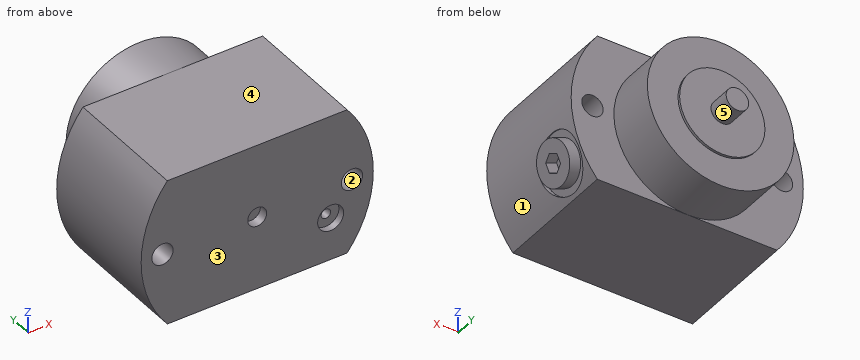
from build123d import *

# Parameters (mm, degrees)
EXTRUDE1_DEPTH     = 53
HOLE1_D            = 9
HOLE1_DEPTH        = 53
SKETCH5_R          = 4
CUT_EXTRUDE1_DEPTH = 4
SKETCH6_R          = 5.5
CUT_EXTRUDE2_DEPTH = 3
SKETCH7_R          = 2
CUT_EXTRUDE3_DEPTH = 33
CUT_EXTRUDE4_DEPTH = 5


with BuildPart() as part:
    # Sketch1 → Extrude1 (new body)
    with BuildSketch(Plane(origin=(0, 0, 0), x_dir=(1, 0, 0), z_dir=(0, 1, 0))):
        with BuildLine():
            Line((-37.947331922, 31), (37.947331922, 31))
            ThreePointArc((37.947331922, 31), (49, 0), (37.947331922, -31))
            Line((37.947331922, -31), (-37.947331922, -31))
            ThreePointArc((-37.947331922, -31), (-49, 0), (-37.947331922, 31))
        make_face()
    extrude(amount=EXTRUDE1_DEPTH)

    # Sketch2 → Revolve1 (revolve)
    with BuildSketch(Plane.XY, mode=Mode.PRIVATE) as revolve1_sk:
        Polygon((0, 84.5), (-4.75, 84.5), (-4.75, 75), (-18, 75), (-18, 74), (-30.95, 74), (-30.95, 53), (0, 53), align=None)
    revolve(revolve1_sk.sketch.rotate(Axis((0, 0, 0), (0, 1, 0)), 270), axis=Axis((0, 0, 0), (0, 1, 0)))  # turned: the seam where the file's is

    # Hole1
    with Locations(Plane(origin=(0, 53, 0), x_dir=(-1, 0, 0), z_dir=(0, 1, 0))):
        with Locations((40, 0), (-40, 0)):
            Hole(HOLE1_D / 2, depth=HOLE1_DEPTH)

    # Sketch5 → Cut-Extrude1 (cut)
    with BuildSketch(Plane.XZ):
        with Locations(Location((0, 0, 0), (0, 0, 270))):  # turned: the seam where the file's is
            Circle(SKETCH5_R)
    extrude(amount=-CUT_EXTRUDE1_DEPTH, mode=Mode.SUBTRACT)

    # Sketch6 → Cut-Extrude2 (cut)
    with BuildSketch(Plane.XZ):
        with Locations(Location((31, -13, 0), (0, 0, 270))):  # turned: the seam where the file's is
            Circle(SKETCH6_R)
    extrude(amount=-CUT_EXTRUDE2_DEPTH, mode=Mode.SUBTRACT)

    # Sketch7 → Cut-Extrude3 (cut)
    with BuildSketch(Plane.XZ.offset(-3)):
        with Locations(Location((31, -13, 0), (0, 0, 270))):  # turned: the seam where the file's is
            Circle(SKETCH7_R)
    extrude(amount=-CUT_EXTRUDE3_DEPTH, mode=Mode.SUBTRACT)

    # Sketch8 → Cut-Revolve1 (revolve, cut)
    with BuildSketch(Plane(origin=(0, 0, 0), x_dir=(0.920504853, 0, -0.390731128), z_dir=(0.390731128, 0, 0.920504853)), mode=Mode.PRIVATE) as cut_revolve1_sk:
        Polygon((49, 28), (47, 28), (47, 33.4215), (45.517364509, 34.2775), (32, 34.2775), (32, 40), (49, 40), align=None)
    revolve(cut_revolve1_sk.sketch.rotate(Axis((47.484793311, 40, -20.156098913), (-0.920504853, 0, 0.390731128)), 270), axis=Axis((47.484793311, 40, -20.156098913), (-0.920504853, 0, 0.390731128)), mode=Mode.SUBTRACT)  # turned: the seam where the file's is

    # Sketch9 → Revolve2 (revolve)
    with BuildSketch(Plane(origin=(0, 0, 0), x_dir=(0.920504853, 0, -0.390731128), z_dir=(0.390731128, 0, 0.920504853)), mode=Mode.PRIVATE) as revolve2_sk:
        Polygon((47, 31), (47, 34.2775), (38, 34.2775), (37, 35.2775), (37, 40), (52, 40), (52, 31), align=None)
    revolve(revolve2_sk.sketch.rotate(Axis((53.930450878, 40, -22.892118224), (-0.920504853, 0, 0.390731128)), 270), axis=Axis((53.930450878, 40, -22.892118224), (-0.920504853, 0, 0.390731128)))  # turned: the seam where the file's is

    # Sketch10 → Cut-Extrude4 (cut)
    with BuildSketch(Plane(origin=(47.86625238, 0, -20.318018681), x_dir=(-0.390731128, 0, -0.920504853), z_dir=(0.920504853, 0, -0.390731128))):
        Polygon((4.041451884, 40), (2.020725942, 43.5), (-2.020725942, 43.5), (-4.041451884, 40), (-2.020725942, 36.5), (2.020725942, 36.5), align=None)
    extrude(amount=-CUT_EXTRUDE4_DEPTH, mode=Mode.SUBTRACT)


solid = part.part
CAD build for the part. Positions are in the model's coordinates, mm. Face numbers are marked on the shaded views. A direction names the side the tool comes from. Round coordinates to 2 decimals unless told otherwise and drop trailing zeros. Order: outer loops, then holes, each group sorted by start corner. A loop starts at its lowest first (then second) coordinate and runs counter-clockwise, first axis right, second up. Notation, with made-up numbers: (82.5, 68) -> (132.5, 68) arc R9 ccw to (132.5, 84) -> close; hole circle Ø1 at (6, 66). An arc over 180 degrees is marked (long way). Write item = value, one per line. Start each with the question number.
(1) Probe line 1 (X direction, y = 19, z = 0.5); line 2 (X direction, y = 81, z = 0); line 3 (Y direction, x = 29, z = 23.5). List the from-to ranges inside material, lowest first. Write a range as [from, to].
(2) Cut at D-D, the plane x = 0. List the corners of the cut face in (y, z), then the cut area to 3 significant figures.
(3) Pin check, flat tips, straight feed: P1, Ø0.8, axis at x = 29.5, z = -12, coming from the -Y side; P2, Ø8, axis at x = 40, z = 0, coming from the -Y side; P3, Ø3, axis at x = 31, z = -13, coming from the -Y side; P4, Ø6, axis at x = 11.5, z = -13.5, coming from the +Y side. Stop position of each tip, or through.
(4) Which spindle directions (+Z, -Z, +X, -X, +Y, -Y) get a long thin tool onto all of the face, cutting with end or side? Do the marked faces 4 and 5. Say none if no direction does.
(5) Pull direction X, two halves, no side cores. Call the marked faces 1, 2 and 3: released by +X, released by -X, zero draft, split by the parting line, or undercut.
(6) Cut at B-B, the plane x = -40. List the corners of the cut face in (y, z), then the cut area to 3 significant figures.
(7) Cut at A-A, the plane z = 0. List the corners of the cut face in (x, y), then the cut area to 3 significant figures.
(8) Cut at C-C, the plane y = 11.5. List the corners of the cut face in (x, z).
Model answer:
q1.line_1 = [-49, -44.47], [-35.53, 35.53], [44.47, 49]
q1.line_2 = [-4.75, 4.75]
q1.line_3 = [0, 53]
q2.outline = (0, -31) -> (53, -31) -> (53, -30.95) -> (74, -30.95) -> (74, -18) -> (75, -18) -> (75, -4.75) -> (84.5, -4.75) -> (84.5, 4.75) -> (75, 4.75) -> (75, 18) -> (74, 18) -> (74, 30.95) -> (53, 30.95) -> (53, 31) -> (0, 31) -> (0, 4) -> (4, 4) -> (4, -4) -> (0, -4) -> close
q2.area = 4,680 mm2
q3.P1 = 3
q3.P2 = through
q3.P3 = 45.48
q3.P4 = 75
q4.face_4 = +Z, +X, -X, +Y, -Y
q4.face_5 = +Y
q5.face_1 = released by +X
q5.face_2 = undercut
q5.face_3 = zero draft
q6.outline = (0, -28.3) -> (53, -28.3) -> (53, -4.5) -> (0, -4.5) -> close; (0, 4.5) -> (53, 4.5) -> (53, 28.3) -> (0, 28.3) -> close
q6.area = 2,520 mm2
q7.outline = (-49, 0) -> (-44.5, 0) -> (-44.5, 53) -> (-49, 53) -> close; (-35.5, 0) -> (-4, 0) -> (-4, 4) -> (4, 4) -> (4, 0) -> (35.5, 0) -> (35.5, 53) -> (30.95, 53) -> (30.95, 74) -> (18, 74) -> (18, 75) -> (4.75, 75) -> (4.75, 84.5) -> (-4.75, 84.5) -> (-4.75, 75) -> (-18, 75) -> (-18, 74) -> (-30.95, 74) -> (-30.95, 53) -> (-35.5, 53) -> close; (44.5, 0) -> (49, 0) -> (49, 53) -> (44.5, 53) -> close
q7.area = 5,630 mm2
q8.outline = (-37.95, -31) -> (37.95, -31) arc R49 ccw to (37.95, 31) -> (-37.95, 31) arc R49 ccw to start; hole circle Ø9 at (-40, 0); hole circle Ø4 at (31, -13); hole circle Ø9 at (40, 0)
